Source: CAD feature listing. Evaluate the final solid. Frame: model axes, mm. A direction names the side the tool comes from. Coordinates: 2 decimals unless noted, no trailing zeros. Write each loop counter-clockwise with the first axis right and the second up, starting at its lowest first coordinate (ties: lowest second). Pieces come first, ordered by that corner, then holes. Notation, with made-up numbers: (45.5, -23) - (80.5, -23) arc R21 cw to (80.5, -15) - close; hole circle Ø10 at (-5, -37). An arc over 180 degrees is marked (long way). One line per question, with ' | ' between items. Start each with the question number.
Q1. Contact query for flat-ended pins moving along their axis: P1, Ø4, axis at x = -19.5, z = 16.5, coming from the -Y side; P2, Ø1.6, axis at x = 26.5, z = 11, coming from the +Y side; P3, Ø1.1, axis at x = 26, y = -5, coming from the +Z side; P4, Ø1.5, axis at y = -49, z = 12, coming from the +X side. Output: stop coordinate, or through.
Q2. Draft query along X for faces 1 (the face through (21.44, -46, 14)), 2 (the face through (-80, -50.816, 11)), 3 (the face through (-197.7, -43, 7)). Return one class per face: +X half, -X half, draft (parallel to the pull), parting line (faces both ways), or undercut.
Q3. Cut plane B-B, the plane x = -2.5. Return loops of the section in (y, z).
Q4. Cut plane D-D, the plane x = -132. Return loops of the section in (y, z), plus the area to 3 significant figures.
Q5. Cut plane A-A, the plane y = -12.5. Return loops of the section in (x, z).
Q6. Cut plane C-C, the plane z = 17.25. Return loops of the section in (x, y), plus the area to 3 significant figures.
Q7. Line query: line 1 (X direction, y = -20, z = 18.5); line 2 (X direction, y = -27.5, z = 1); line 3 (Y direction, x = -177.5, z = 12.5). Output: solid intervals per line, ascending.
Q8. Access query for faces 4 (the face through (-9, 2, 12.5)), 5 (the face through (29.94, -21, 3)), 6 (the face through (-9, -8, 0)), 7 (the face through (-106, -40.816, 5)), 8 (the face through (-80, -48, 1)). Directions: +Z, -Z, +X, -X, +Y, -Y. A direction counts if a zero-diameter tool reaches every point of the face in a straight line with its end or side. Return the directions, or none.
```python
from build123d import *

# Parameters (mm, degrees)
SKETCH2_W           = 100
SKETCH2_H           = 50
BOSS_EXTRUDE1_DEPTH = 20
SHELL1_T            = -5
SKETCH5_W           = 72
SKETCH5_H           = 25
CUT_EXTRUDE1_DEPTH  = 77.995878023
SKETCH6_R           = 1.8
CUT_EXTRUDE2_DEPTH  = 77.995878023
SKETCH7_W           = 6
SKETCH7_H           = 8
CUT_EXTRUDE3_DEPTH  = 4
SKETCH8_W           = 239.14
SKETCH8_H           = 25
BOSS_EXTRUDE2_DEPTH = 5
SKETCH9_W           = 228
SKETCH9_H           = 19
BOSS_EXTRUDE3_DEPTH = 5
SKETCH10_W          = 60
SKETCH10_H          = 13
CUT_EXTRUDE4_DEPTH  = 19
SKETCH11_R          = 1.2
BOSS_EXTRUDE4_DEPTH = 5
SKETCH12_R          = 1.2
BOSS_EXTRUDE5_DEPTH = 5
SKETCH13_R          = 1.2
BOSS_EXTRUDE6_DEPTH = 5
SKETCH14_R          = 1.2
BOSS_EXTRUDE7_DEPTH = 5
FILLET3_R           = 0.5
FILLET4_R           = 0.5
FILLET5_R           = 0.5
FILLET6_R           = 0.5
SKETCH16_W          = 15
SKETCH16_H          = 2
CUT_EXTRUDE5_DEPTH  = 1
SKETCH17_W          = 90
SKETCH17_H          = 2
CUT_EXTRUDE6_DEPTH  = 205.903131616


with BuildPart() as part:
    # Sketch2 → Boss-Extrude1 (new body)
    with BuildSketch(Plane.XY):
        with Locations((-8.560008462, -20.815833959)):
            Rectangle(SKETCH2_W, SKETCH2_H)
    extrude(amount=BOSS_EXTRUDE1_DEPTH)

    # Shell1
    shell1_openings = [part.faces().sort_by_distance(p)[0] for p in [
        (-8.560008462, -20.815833959, 20),
    ]]
    offset(amount=SHELL1_T, openings=shell1_openings, kind=Kind.INTERSECTION)

    # Sketch5 → Cut-Extrude1 (cut, through all)
    with BuildSketch(Plane(origin=(0, 0, 0), x_dir=(-1, 0, 0), z_dir=(0, 0, -1))):
        with Locations((11.560008462, -20.815833959)):
            Rectangle(SKETCH5_W, SKETCH5_H)
    extrude(amount=-CUT_EXTRUDE1_DEPTH, mode=Mode.SUBTRACT)

    # Sketch6 → Cut-Extrude2 (cut, through all)
    with BuildSketch(Plane(origin=(0, 0, 0), x_dir=(-1, 0, 0), z_dir=(0, 0, -1))):
        with Locations((-32.939991538, -20.815833959)):
            Circle(SKETCH6_R)
    extrude(amount=-CUT_EXTRUDE2_DEPTH, mode=Mode.SUBTRACT)

    # Sketch7 → Cut-Extrude3 (cut)
    with BuildSketch(Plane.XY.offset(5)):
        with Locations((32.939991538, -20.815833959)):
            Rectangle(SKETCH7_W, SKETCH7_H)
    extrude(amount=-CUT_EXTRUDE3_DEPTH, mode=Mode.SUBTRACT)

    # Sketch8 → Boss-Extrude2 (add)
    with BuildSketch(Plane.XZ.offset(45.815833959)):
        with Locations((-78.130008462, 7.5)):
            Rectangle(SKETCH8_W, SKETCH8_H)
    extrude(amount=-BOSS_EXTRUDE2_DEPTH)

    # Sketch9 → Boss-Extrude3 (add)
    with BuildSketch(Plane.XZ.offset(45.815833959)):
        with Locations((-78.130008462, 10.5)):
            Rectangle(SKETCH9_W, SKETCH9_H)
    extrude(amount=BOSS_EXTRUDE3_DEPTH)

    # Sketch10 → Cut-Extrude4 (cut)
    with BuildSketch(Plane(origin=(0, -40.815833959, 0), x_dir=(1, 0, 0), z_dir=(0, 1, 0))):
        with Locations((-8.560008462, -13.5)):
            Rectangle(SKETCH10_W, SKETCH10_H)
    extrude(amount=-CUT_EXTRUDE4_DEPTH, mode=Mode.SUBTRACT)

    # Sketch11 → Boss-Extrude4 (add)
    with BuildSketch(Plane.XY.offset(5)):
        with Locations((-49.420008462, -4.775833959)):
            Circle(SKETCH11_R)
    extrude(amount=BOSS_EXTRUDE4_DEPTH)

    # Sketch12 → Boss-Extrude5 (add)
    with BuildSketch(Plane.XY.offset(5)):
        with Locations((25.579991538, -4.775833959)):
            Circle(SKETCH12_R)
    extrude(amount=BOSS_EXTRUDE5_DEPTH)

    # Sketch13 → Boss-Extrude6 (add)
    with BuildSketch(Plane.XY.offset(5)):
        with Locations((-49.420008462, -35.775833959)):
            Circle(SKETCH13_R)
    extrude(amount=BOSS_EXTRUDE6_DEPTH)

    # Sketch14 → Boss-Extrude7 (add)
    with BuildSketch(Plane.XY.offset(5)):
        with Locations((25.579991538, -35.775833959)):
            Circle(SKETCH14_R)
    extrude(amount=BOSS_EXTRUDE7_DEPTH)

    # Fillet3
    fillet3_edges = [part.edges().sort_by_distance(p)[0] for p in [
        (-50.620008462, -35.775833959, 10),
    ]]
    fillet(fillet3_edges, radius=FILLET3_R)

    # Fillet4
    fillet4_edges = [part.edges().sort_by_distance(p)[0] for p in [
        (-50.620008462, -4.775833959, 10),
    ]]
    fillet(fillet4_edges, radius=FILLET4_R)

    # Fillet5
    fillet5_edges = [part.edges().sort_by_distance(p)[0] for p in [
        (24.379991538, -4.775833959, 10),
    ]]
    fillet(fillet5_edges, radius=FILLET5_R)

    # Fillet6
    fillet6_edges = [part.edges().sort_by_distance(p)[0] for p in [
        (24.379991538, -35.775833959, 10),
    ]]
    fillet(fillet6_edges, radius=FILLET6_R)

    # Sketch16 → Cut-Extrude5 (cut)
    with BuildSketch(Plane(origin=(0, -40.815833959, 0), x_dir=(1, 0, 0), z_dir=(0, 1, 0))):
        with Locations((-46.060008462, -11.5)):
            Rectangle(SKETCH16_W, SKETCH16_H)
        with Locations((28.939991538, -11.5)):
            Rectangle(SKETCH16_W, SKETCH16_H)
    extrude(amount=-CUT_EXTRUDE5_DEPTH, mode=Mode.SUBTRACT)

    # Sketch17 → Cut-Extrude6 (cut, through all)
    with BuildSketch(Plane.XZ.offset(0.815833959)):
        with Locations((-8.560008462, 11.5)):
            Rectangle(SKETCH17_W, SKETCH17_H)
    extrude(amount=-CUT_EXTRUDE6_DEPTH, mode=Mode.SUBTRACT)


solid = part.part
```
Reply:
1) P1: stops at y = -0.82 | P2: stops at y = 4.18 | P3: stops at z = 10 | P4: stops at x = 35.87
2) face 1: undercut | face 2: draft | face 3: -X half
3) outline: (-50.82, 1) - (-45.82, 1) - (-45.82, -5) - (-40.82, -5) - (-40.82, 0) - (-33.32, 0) - (-33.32, 5) - (-40.82, 5) - (-40.82, 7) - (-50.82, 7) - close; (-8.32, 0) - (4.18, 0) - (4.18, 10.5) - (-0.82, 10.5) - (-0.82, 5) - (-8.32, 5) - close; (-0.82, 12.5) - (4.18, 12.5) - (4.18, 20) - (-0.82, 20) - close
4) outline: (-50.82, 1) - (-45.82, 1) - (-45.82, -5) - (-40.82, -5) - (-40.82, 20) - (-50.82, 20) - close | area: 220 mm^2
5) outline: (-58.56, 0) - (-47.56, 0) - (-47.56, 5) - (-53.56, 5) - (-53.56, 20) - (-58.56, 20) - close; (24.44, 0) - (41.44, 0) - (41.44, 20) - (36.44, 20) - (36.44, 5) - (24.44, 5) - close
6) outline: (-197.7, -45.82) - (-192.13, -45.82) - (-192.13, -50.82) - (-38.56, -50.82) - (-38.56, -40.82) - (-53.56, -40.82) - (-53.56, -0.82) - (36.44, -0.82) - (36.44, -40.82) - (21.44, -40.82) - (21.44, -50.82) - (35.87, -50.82) - (35.87, -45.82) - (41.44, -45.82) - (41.44, 4.18) - (-58.56, 4.18) - (-58.56, -40.82) - (-197.7, -40.82) - close | area: 2,640 mm^2
7) line 1: x = -58.56 to -53.56, 36.44 to 41.44 | line 2: x = -58.56 to -47.56, 24.44 to 41.44 | line 3: y = -50.82 to -40.82
8) face 4: +Y | face 5: +Z | face 6: -Z, +X, -X, +Y | face 7: -Z, -X, +Y | face 8: -Z, +X, -X, -Y
